Geometry: see drawing. Coordinates: mm, zero at the bounding-box minimum. Give positions to 0.01 mm unless a question says otherwise; leave off trailing zeros. Loops run counter-clockwise (first coordinate to the right, second up) from the corner with the lowest first, then second, coordinate; pieces in that order, holes last. Notation, with made-up numbers: (21, 15) -> (54, 15) arc R38 cw to (54, 53) -> close; hole circle Ø9 at (33, 11). An arc over 180 degrees is marked (long way). Use CSV: the item, a comma, the result in double quotes.
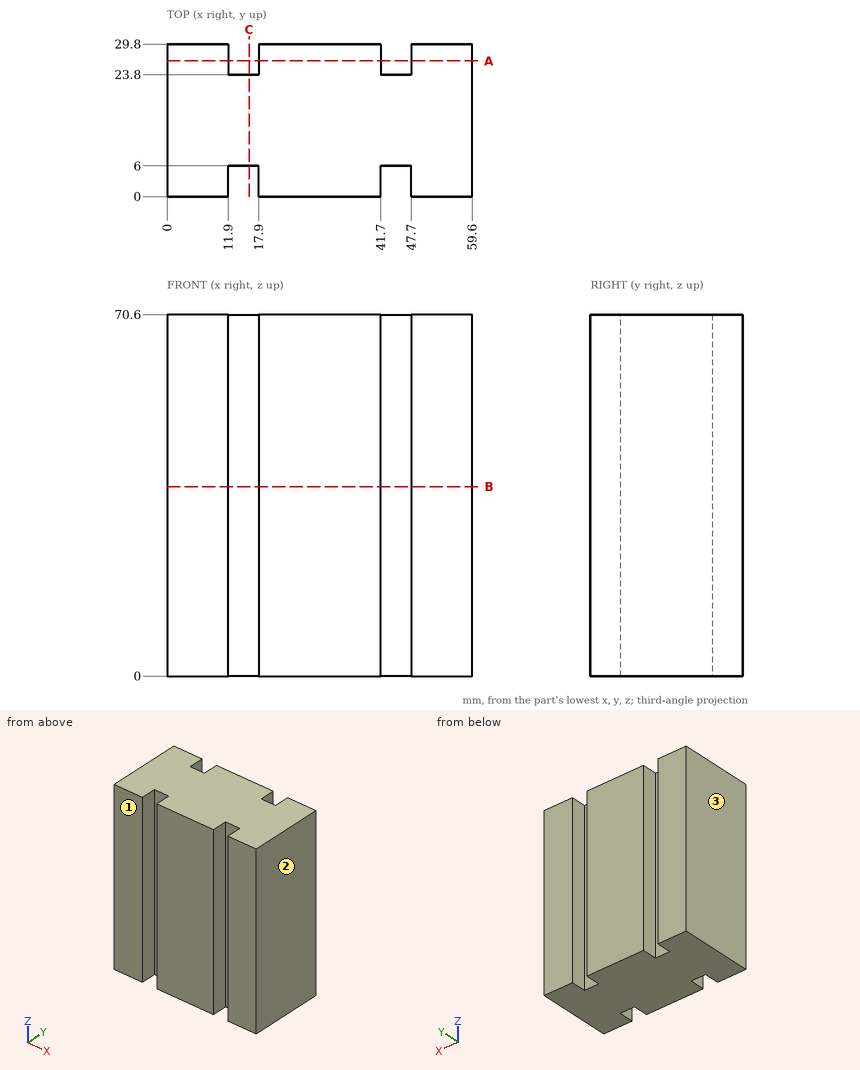
1) Ray query, line 1 (X direction, y = 28.5, z = 33); line 2 (Y direction, x = 12.5, z = 64.5). Return the intervals inside material, ascending.
From the geometry:
line 1,"x = 0 to 11.9, 17.9 to 41.7, 47.7 to 59.6"
line 2,"y = 6 to 23.8"
2) Section query C-C (x = 16). Return loops of the section in (y, z).
From the geometry:
outline,"(6, 0) -> (23.8, 0) -> (23.8, 70.6) -> (6, 70.6) -> close"
3) Section query B-B (z = 37). Return loops of the section in (x, y).
From the geometry:
outline,"(0, 0) -> (11.9, 0) -> (11.9, 6) -> (17.9, 6) -> (17.9, 0) -> (41.7, 0) -> (41.7, 6) -> (47.7, 6) -> (47.7, 0) -> (59.6, 0) -> (59.6, 29.8) -> (47.7, 29.8) -> (47.7, 23.8) -> (41.7, 23.8) -> (41.7, 29.8) -> (17.9, 29.8) -> (17.9, 23.8) -> (11.9, 23.8) -> (11.9, 29.8) -> (0, 29.8) -> close"
4) Mould query, pull axis X, two halves, no side actions, for the marked faces 1, 2 and 3. Classes: pulls with the +X half, pulls with the -X half, needs draft (parallel to the pull), parting line crosses it, or undercut.
From the geometry:
face 1,"needs draft"
face 2,"pulls with the +X half"
face 3,"pulls with the -X half"
5) Section query A-A (y = 26.5). Return loops of the section in (x, z), then the cut area to 3 significant figures.
From the geometry:
outline,"(0, 0) -> (11.9, 0) -> (11.9, 70.6) -> (0, 70.6) -> close; (17.9, 0) -> (41.7, 0) -> (41.7, 70.6) -> (17.9, 70.6) -> close; (47.7, 0) -> (59.6, 0) -> (59.6, 70.6) -> (47.7, 70.6) -> close"
area,"3,360 mm^2"
6) Contact query for flat-ended pins moving along their axis: pin 1 (3 mm diameter, centred on x = 44.5, z = 39, fed in from +Y); pin 2 (5 mm diameter, centred on x = 15, z = 28, fed in from -Y). Output: stop coordinate, or through.
From the geometry:
pin 1,"stops at y = 23.8"
pin 2,"stops at y = 6"
